CAD build for the part. Positions are in the model's coordinates, mm. Face numbers are marked on the shaded views. Round coordinates to 2 decimals unless told otherwise and drop trailing zeros. Write each loop counter-clockwise with the first axis right and the second up, starting at its lowest first coordinate (ties: lowest second). Pieces come first, ordered by that corner, then holes. Notation, with made-up numbers: (80, -7.5) - (111, -7.5) arc R19 ccw to (111, 11.5) - close; hole circle Ø11 at (85, 72). An arc over 180 degrees is marked (long way). Answer in a Markdown table with one row per item.
```python
from build123d import *

# Parameters (mm, degrees)
F6_W     = 508
F6_H     = 508
F7_DEPTH = 25.4
F8_W     = 19.05
F8_H     = 152.4
F9_DEPTH = 25.4
F0_R     = 38.1
F2_DEPTH = 3.175
F3_R     = 38.1
F5_D     = 3.175
F5_DEPTH = 63.5
F5_TIP   = 0.9538662327


with BuildPart() as f7:
    # F6 (on Top) → F7 (new body)
    with BuildSketch(Plane.XY):
        Rectangle(F6_W, F6_H)
    extrude(amount=F7_DEPTH)

    # F8 (on face) → F9 (cut)
    with BuildSketch(Plane.XY.offset(25.4)):
        with Locations((-76.2, 177.8)):
            Rectangle(F8_W, F8_H)
    extrude(amount=-F9_DEPTH, mode=Mode.SUBTRACT)

    # F0
    f0_edges = [f7.edges().sort_by_distance(p)[0] for p in [
        (254, -254, 12.7),
        (254, 254, 12.7),
        (-254, 254, 12.7),
        (-254, -254, 12.7),
    ]]
    fillet(f0_edges, radius=F0_R)

    # F1 (on face) → F2 (cut)
    with BuildSketch(Plane.XY.offset(25.4)):
        Polygon((190.5, 190.5), (0, 190.5), (0, 0), (-190.5, 0), (-190.5, -190.5), (190.5, -190.5), align=None)
    extrude(amount=-F2_DEPTH, mode=Mode.SUBTRACT)

    # F3
    f3_edges = [f7.edges().sort_by_distance(p)[0] for p in [
        (0, 0, 23.8125),
        (0, 190.5, 23.8125),
        (190.5, 190.5, 23.8125),
        (-190.5, -190.5, 23.8125),
        (190.5, -190.5, 23.8125),
        (-190.5, 0, 23.8125),
    ]]
    fillet(f3_edges, radius=F3_R)

    # F5
    with Locations(Plane(origin=(0, 254, 0), x_dir=(-1, 0, 0), z_dir=(0, 1, 0))):
        with Locations((-12.7, 12.7), (165.1, 12.7)):
            Hole(F5_D / 2, depth=F5_DEPTH)
            with Locations((0, 0, -(F5_DEPTH + F5_TIP / 2))):  # 118° drill point
                Cone(0, F5_D / 2, F5_TIP, mode=Mode.SUBTRACT)


solid = f7.part
```
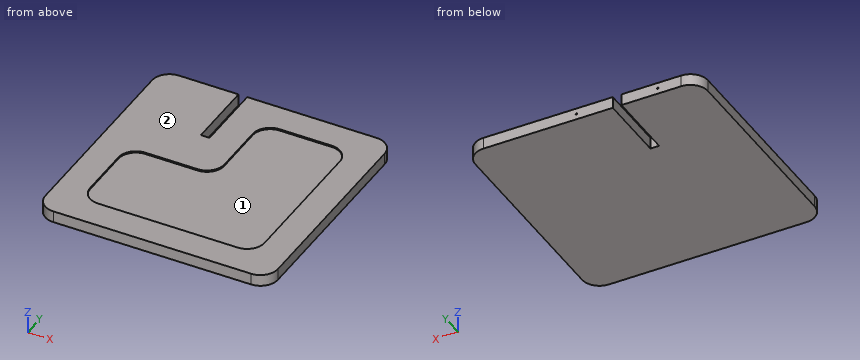
Q1. Drill centre lines: line 1 (X direction, y = 150.5, z = 23.25) (3 decimals); line 2 (X direction, y = 204.5, z = 12.7) (1 decimal); line 3 (Z direction, x = 12.7, y = 222.5). Where is each one in solid material? Low to high.
Computed:
| item | result |
|---|---|
| line 1 | x = -254 to -85.725, -66.675 to 0, 190.5 to 254 |
| line 2 | x = -254 to -166.7, -163.5 to -85.7, -66.7 to 11.1, 14.3 to 254 |
| line 3 | z = 0 to 11.11, 14.29 to 25.4 |
Q2. Saw through at C-C on y = -95.5. List the corners of the cut face in (x, z) (3 decimals).
Computed:
| item | result |
|---|---|
| outline | (-254, 0) - (254, 0) - (254, 25.4) - (190.5, 25.4) - (190.5, 22.225) - (-190.5, 22.225) - (-190.5, 25.4) - (-254, 25.4) - close |
Q3. Flat gauge pins, fed straight in: pin 1 (1 mm diameter, centred on x = -126.5, y = 163, fed in from -Z); pin 2 (5.5 mm diameter, centred on x = -79, z = 10.5, fed in from +Y); pin 3 (1.9 mm diameter, centred on x = 12.7, z = 12.7, fed in from +Y). Where does each tip first touch, or does it go through?
Computed:
| item | result |
|---|---|
| pin 1 | stops at z = 0 |
| pin 2 | stops at y = 101.6 |
| pin 3 | stops at y = 190.12 |
Q4. Saw through at B-B on z = 4.5. List the corners of the cut face in (x, y) (3 decimals).
Computed:
| item | result |
|---|---|
| outline | (-254, -215.9) arc R38.1 ccw to (-215.9, -254) - (215.9, -254) arc R38.1 ccw to (254, -215.9) - (254, 215.9) arc R38.1 ccw to (215.9, 254) - (-66.675, 254) - (-66.675, 101.6) - (-85.725, 101.6) - (-85.725, 254) - (-215.9, 254) arc R38.1 ccw to (-254, 215.9) - close |
Q5. Pull direction Y, two halves, no side cores. Call the marked faces 1 and 2: released by +Y, released by -Y, zero draft, split by the parting line, or undercut.
Computed:
| item | result |
|---|---|
| face 1 | undercut |
| face 2 | zero draft |
Q6. Saw through at A-A on y = 143. List the corners of the cut face in (x, z) (3 decimals).
Computed:
| item | result |
|---|---|
| outline | (-254, 0) - (-85.725, 0) - (-85.725, 25.4) - (-254, 25.4) - close; (-66.675, 0) - (254, 0) - (254, 25.4) - (190.5, 25.4) - (190.5, 22.225) - (0, 22.225) - (0, 25.4) - (-66.675, 25.4) - close |
